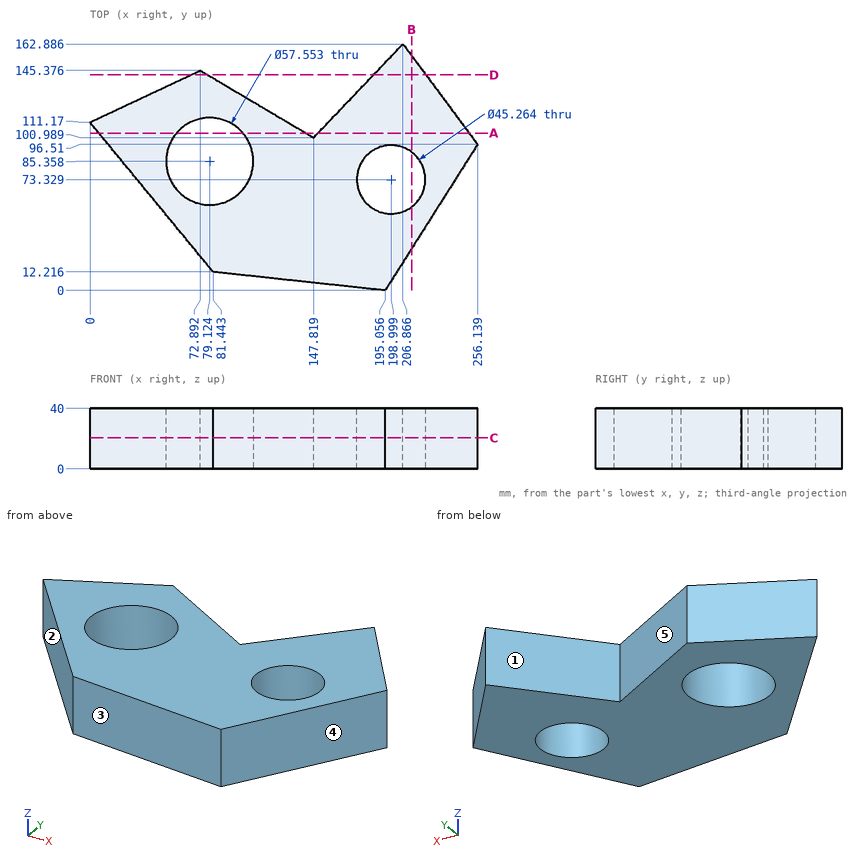
Answer from the drawing. Dimensions are ordinates in mm from the lowest x, y and z of the part. A direction names the side the tool comes from. Give positions to 0.01 mm unless a question says otherwise; leave off trailing zeros. Order: outer loops, then holes, each group sorted by start corner. A loop starts at its lowest first (then second) coordinate and runs counter-clockwise, first axis right, second up. Notation, with made-up numbers: (25, -8.5) - (67, -8.5) arc R5 ccw to (67, -1.5) - close; hole circle Ø7 at (-35, 77). An arc over 180 degrees is marked (long way). Use one line per item in the form item = value.
1) Find section D-D on y = 142.5. Determine the outline of the cut face in (x, z), and give its area (3 significant figures).
Verdict:
outline = (66.76, 0) - (77.75, 0) - (77.75, 40) - (66.76, 40) - close; (187.42, 0) - (222, 0) - (222, 40) - (187.42, 40) - close
area = 1,820 mm^2
2) Consider probe 1 along X at (y, z) = (93, 37) (1 decimal); probe 2 along X at (y, z) = (90.5, 10.5) (1 decimal); probe 3 along Y at (x, z) = (83.5, 28.5) (1 decimal). Determine where each line is inside the solid, lowest interval first. Write a range as [from, to].
Verdict:
probe_1 = [15, 51.4], [106.9, 187.8], [210.2, 253.9]
probe_2 = [17, 50.8], [107.4, 184.3], [213.7, 252.3]
probe_3 = [12, 56.9], [113.8, 139.1]
3) Each of these flat-tipped pins is pushed along its axis until it touches: pin 1 (4 mm diameter, centred on x = 41, y = 124.5, fed in from -Z); pin 2 (2 mm diameter, centred on y = 97, z = 4.5, fed in from -X); pin 3 (3 mm diameter, centred on y = 132.5, z = 23.5, fed in from +X) (1 decimal); pin 4 (1.5 mm diameter, centred on y = 58.5, z = 20.5, fed in from -X). Where does it stop, or does it pass through?
Verdict:
pin_1 = 0
pin_2 = 10.84
pin_3 = 230.5
pin_4 = 42.73
4) Find section A-A on y = 104. Determine the outline of the cut face in (x, z) (1 decimal).
Verdict:
outline = (5.9, 0) - (57.2, 0) - (57.2, 40) - (5.9, 40) - close; (101, 0) - (142.7, 0) - (142.7, 40) - (101, 40) - close; (150.7, 0) - (250.6, 0) - (250.6, 40) - (150.7, 40) - close
5) Find section C-C on z = 20.5. Determine the outline of the cut face in (x, y) (1 decimal).
Verdict:
outline = (0, 111.2) - (81.4, 12.2) - (195.1, 0) - (256.1, 96.5) - (206.9, 162.9) - (147.8, 101) - (72.9, 145.4) - close; hole circle Ø57.6 at (79.1, 85.4); hole circle Ø45.3 at (199, 73.3)
6) For the marked faces 1 and 2, determine the directions among +Z, -Z, +X, -X, +Y, -Y from which every point of the face is accessible in a straight line to the end or side of a thin tool.
Verdict:
face_1 = +Z, -Z, +Y
face_2 = +Z, -Z, -X, -Y
7) Find section B-B on x = 212.5. Determine the outline of the cut face in (y, z) (1 decimal), and give its area (3 significant figures).
Verdict:
outline = (27.6, 0) - (55.2, 0) - (55.2, 40) - (27.6, 40) - close; (91.5, 0) - (155.3, 0) - (155.3, 40) - (91.5, 40) - close
area = 3,660 mm^2
8) The mould has two halves that part along X. Classify the marked faces 3, 4 and 5: released by +X, released by -X, zero draft, split by the parting line, or undercut.
Verdict:
face_3 = released by -X
face_4 = released by +X
face_5 = undercut
